Study the drawing (mm; zero at the part's minimum x, y, z) and answer. Round coordinates to 2 decimals unless told otherwise and drop trailing zeros. Write each loop counter-clockwise with the first axis right and the second up, starting at its lowest first coordinate (ties: lowest second). Pieces come first, ordered by that corner, then holes.
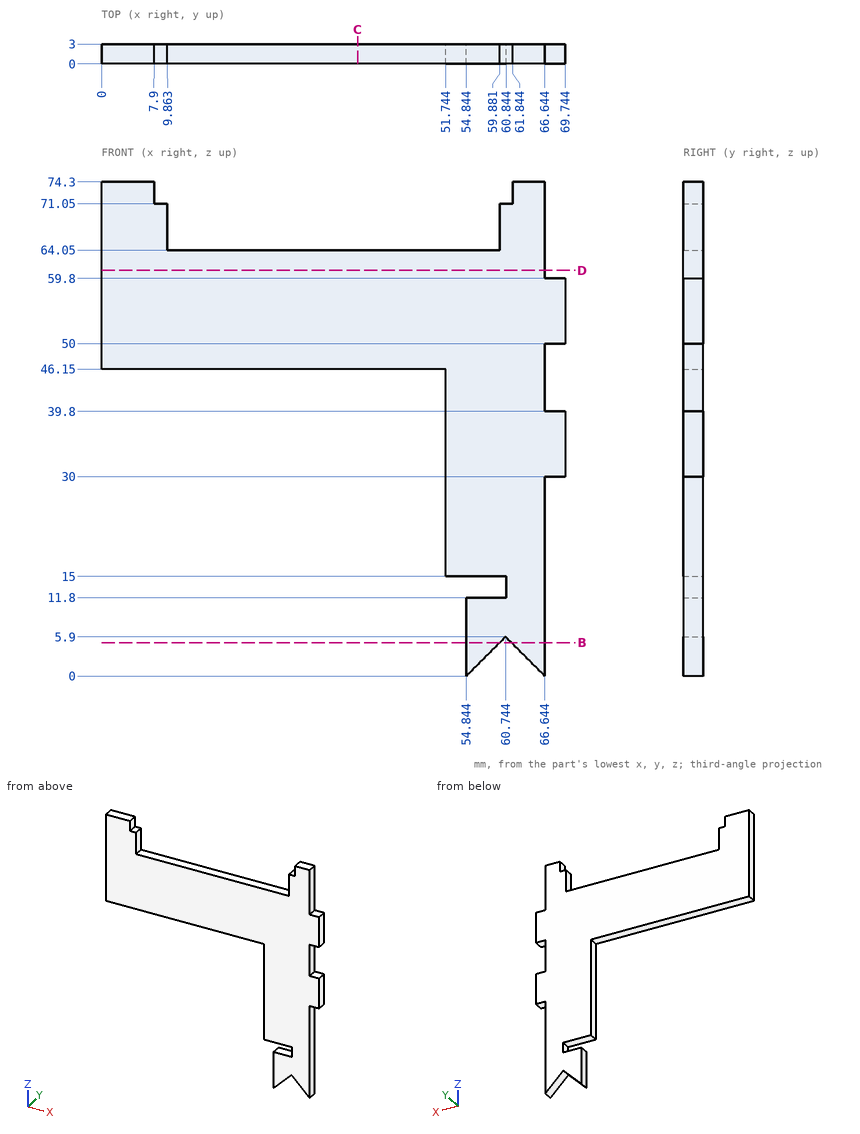
Q1. Find section D-D (z = 61). Determine the outline of the cut face in (x, y) (1 decimal), plus the area to 3 significant figures.
Q2. Find section C-C (x = 38.5). Determine the outline of the cut face in (y, z), plus the area to 3 significant figures.
Q3. Given pin 1 (1.5 mm diameter, centred on x = 57.5, y = 2, fed in from +Z); pin 2 (5 mm diameter, centred on x = 56.5, z = 44, fed in from -Y); pin 3 (1.5 mm diameter, centred on x = 38, y = 2, fed in from -Z); pin 4 (0.9 mm diameter, centred on y = 1.5, z = 67, fed in from +X), each flat-ended and moving along its own axis, determine where each tip first touches the part or whether it passes through.
Q4. Find section B-B (z = 5). Determine the outline of the cut face in (x, y) (1 decimal).
Q5. Find the intervals of material crossed by L1, parallel to Z at x = 34, y = 2.65; L2, parallel to X at y = 0.35, z = 31.5 (1 decimal); L3, parallel to Z at x = 4, y = 0.8, in increasing order.
Report:
1. outline: (0, 0) - (66.6, 0) - (66.6, 3) - (0, 3) - close
1. area: 200 mm2
2. outline: (0, 46.15) - (3, 46.15) - (3, 64.05) - (0, 64.05) - close
2. area: 53.7 mm2
3. pin 1: stops at z = 64.05
3. pin 2: stops at y = 0
3. pin 3: stops at z = 46.15
3. pin 4: stops at x = 66.64
4. outline: (54.8, 0) - (59.8, 0) - (59.8, 3) - (54.8, 3) - close; (61.6, 0) - (66.6, 0) - (66.6, 3) - (61.6, 3) - close
5. L1: z = 46.15 to 64.05
5. L2: x = 51.7 to 69.7
5. L3: z = 46.15 to 74.3
